Build history of the part. All positions in model axes, mm. Face numbers are marked on the shaded views. A direction names the side the tool comes from. Coordinates: 2 decimals unless noted, no trailing zeros. Write each loop counter-clockwise with the first axis right and the second up, starting at its lowest first coordinate (ties: lowest second). Pieces come first, ordered by that corner, then holes.
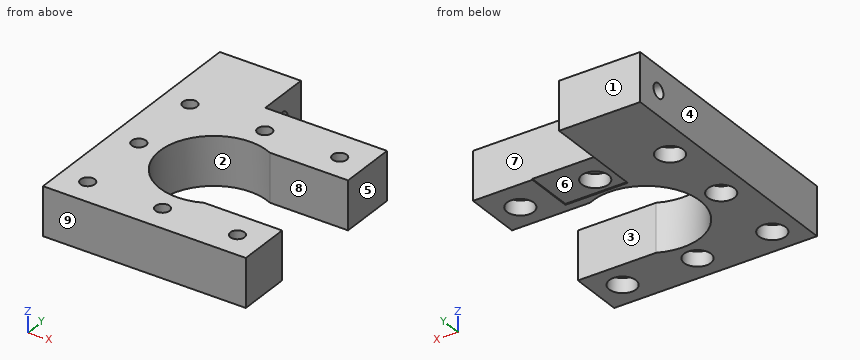
from build123d import *

# Parameters (mm, degrees)
SKETCH054_R          = 1.475
PAD016_DEPTH         = 10
SKETCH055_R          = 2.76
POCKET034_DEPTH      = 3
SKETCH056_R          = 11.1
POCKET035_DEPTH      = 10.001
POCKET035_DEPTH_BACK = 0.001
PAD017_DEPTH         = 10
SKETCH058_R          = 1.5
POCKET036_DEPTH      = 21.001
SKETCH059_W          = 12.9
SKETCH059_H          = 10.2
POCKET037_DEPTH      = 0.2


with BuildPart() as part:
    # Sketch054 → Pad016 (new body)
    with BuildSketch(Plane.XY):
        with BuildLine():
            Line((-21, 21), (21, 21))
            Line((21, 21), (21, 10))
            Line((21, 10), (0, 10))
            ThreePointArc((0, 10), (-10, 0), (0, -10))
            Line((21, -10), (0, -10))
            Line((21, -21), (21, -10))
            Line((21, -21), (-21, -21))
            Line((-21, -21), (-21, 21))
        make_face()
        with Locations((-15.5, 15.5)):
            Circle(SKETCH054_R, mode=Mode.SUBTRACT)
        with Locations((15.5, 15.5)):
            Circle(SKETCH054_R, mode=Mode.SUBTRACT)
        with Locations((-15.5, -15.5)):
            Circle(SKETCH054_R, mode=Mode.SUBTRACT)
        with Locations((15.5, -15.5)):
            Circle(SKETCH054_R, mode=Mode.SUBTRACT)
        with Locations((-15.5, 0)):
            Circle(SKETCH054_R, mode=Mode.SUBTRACT)
        with Locations((0, 15.5)):
            Circle(SKETCH054_R, mode=Mode.SUBTRACT)
        with Locations((0, -15.5)):
            Circle(SKETCH054_R, mode=Mode.SUBTRACT)
    extrude(amount=PAD016_DEPTH)

    # Sketch055 → Pocket034 (cut)
    with BuildSketch(Plane.XY):
        with Locations((-15.5, 15.5)):
            Circle(SKETCH055_R)
        with Locations((15.5, 15.5)):
            Circle(SKETCH055_R)
        with Locations((-15.5, -15.5)):
            Circle(SKETCH055_R)
        with Locations((15.5, -15.5)):
            Circle(SKETCH055_R)
        with Locations((-15.5, 0)):
            Circle(SKETCH055_R)
        with Locations((0, 15.5)):
            Circle(SKETCH055_R)
        with Locations((0, -15.5)):
            Circle(SKETCH055_R)
    extrude(amount=POCKET034_DEPTH, mode=Mode.SUBTRACT)

    # Sketch056 (on Face5 of Pocket034) → Pocket035 (cut, two sides)
    with BuildSketch(Plane.XY.offset(10)) as pocket035_sk:
        Circle(SKETCH056_R)
    extrude(amount=-POCKET035_DEPTH, mode=Mode.SUBTRACT)
    extrude(pocket035_sk.sketch, amount=POCKET035_DEPTH_BACK, mode=Mode.SUBTRACT)

    # Sketch057 → Pad017 (join)
    with BuildSketch(Plane.XY):
        Polygon((-4.2, 21.8), (-4.2, 32.6), (-21, 32.6), (-21, 21), (21, 21), (21, 21.8), align=None)
    extrude(amount=PAD017_DEPTH)

    # Sketch058 → Pocket036 (cut, through all)
    with BuildSketch(Plane.YZ):
        with Locations((27.05, 5)):
            Circle(SKETCH058_R)
    extrude(amount=-POCKET036_DEPTH, mode=Mode.SUBTRACT)

    # Sketch059 → Pocket037 (cut)
    with BuildSketch(Plane.XY):
        with Locations((2.25, 16.9)):
            Rectangle(SKETCH059_W, SKETCH059_H)
    extrude(amount=POCKET037_DEPTH, mode=Mode.SUBTRACT)


with BuildPart() as part_1:
    # Body011 placement: moved
    add(part.part.moved(Location((0, 0, -30))))


solid = part_1.part
(1) Slice it at D-D, the plane x = -9.5. List the corners of the cut face in (y, z), and give its area (3 significant figures).
(2) Slice it at A-A, the plane x = -15.5. Give the number of separate pieces and of enclosed holes in the cut face, and give its area (3 significant figures).
(3) Two-plate mould, pull along Y, no slides. Class the marked faces 1, 2, 3 and 4: pulls with the +Y half, pulls with the -Y half, needs draft (parallel to the pull), parting line crosses it, or undercut.
(4) Probe L1, parallel to Y at x = -15.5, z = -28.8; L2, parallel to X at y = 15.5, z = -25.5 (3 decimals); L3, parallel to Y at x = 15.5, z = -28.15. List the from-to ranges inside material, lowest first.
(5) Slice it at C-C, the plane z = -21. List the corners of the cut face in (x, y) (3 decimals).
(6) 3-axis set-ups, long thin cutter, end or side, ignore diameter. For the marked faces 5, 6, 7, 8 and 9: which of +Z, -Z, +X, -X, +Y, -Y reach the whole face in a straight line?
(7) Flat gauge pins, fed straight in: P1, Ø3, axis at x = 5, y = 16.5, coming from the -Z side; P2, Ø4.5, axis at x = 0, y = 15.5, coming from the -Z side; P3, Ø4, axis at y = 0, z = -27.5, coming from the +X side; P4, Ø2.5, axis at x = 0, y = 15.5, coming from the -Z side. Where does each tip first touch, or does it go through?
Results:
1. outline: (-21, -30) - (-5.74, -30) - (-5.74, -20) - (-21, -20) - close; (5.74, -30) - (32.6, -30) - (32.6, -20) - (5.74, -20) - close; hole circle Ø3 at (27.05, -25)
1. area: 414 mm2
2. separate pieces: 4
2. enclosed holes: 1
2. area: 417 mm2
3. face 1: pulls with the +Y half
3. face 2: undercut
3. face 3: undercut
3. face 4: needs draft
4. L1: y = -21 to -18.26, -12.74 to -2.76, 2.76 to 12.74, 18.26 to 32.6
4. L2: x = -21 to -16.975, -14.025 to -1.475, 1.475 to 14.025, 16.975 to 21
4. L3: y = -21 to -18.26, -12.74 to -10, 10 to 12.74, 18.26 to 21.8
5. outline: (-21, -21) - (21, -21) - (21, -10) - (4.818, -10) arc R11.1 cw (long way) to (4.818, 10) - (21, 10) - (21, 21.8) - (-4.2, 21.8) - (-4.2, 32.6) - (-21, 32.6) - close; hole circle Ø2.95 at (-15.5, -15.5); hole circle Ø2.95 at (-15.5, 0); hole circle Ø2.95 at (-15.5, 15.5); hole circle Ø2.95 at (0, -15.5); hole circle Ø2.95 at (0, 15.5); hole circle Ø2.95 at (15.5, -15.5); hole circle Ø2.95 at (15.5, 15.5)
6. face 5: +Z, -Z, +X, +Y, -Y
6. face 6: -Z, +Y
6. face 7: +Z, -Z, +X, +Y
6. face 8: +Z, -Z, +X
6. face 9: +Z, -Z, +X, -X, -Y
7. P1: stops at z = -29.8
7. P2: stops at z = -27
7. P3: stops at x = -10.92
7. P4: passes through
